Check sheet for the modelled part. Datum: model origin and axes. Units: mm. Face numbers are marked on the shaded views. A direction names the side the tool comes from. Coordinates: 2 decimals unless noted, no trailing zeros. Write each loop counter-clockwise with the first axis right and the second up, starting at its lowest first coordinate (ties: lowest second). Pieces come first, ordered by that corner, then holes. Notation, with made-up numbers: M -15,-4.5 L -10,-4.5 A17 cw -10,7.5 Z; hole C -32.5,9.5 d2. An arc over 180 degrees is marked long. Answer as CSV lines item,"result". Start each with the question number.
Q1. Sectioned sample at C-C, the plane x = -5. Record the cut outline in (y, z) (3 decimals), then the cut area to 3 significant figures.
Q2. Sectioned sample at A-A, the plane y = 10.75. Record the cut outline in (x, z) (1 decimal).
Q3. Depth check by flat-ended pin: pin 1 Ø2.5 at (x, y) = (33, 9.5) entering from -Z; pin 2 Ø3.5 at (x, z) = (-33.5, 1) entering from -Y; pin 3 Ø3 at (x, z) = (-20, 2) entering from +Y (3 decimals); pin 4 Ø2.5 at (y, z) = (10, 0) entering from -X. Enter the tip coordinate at first touch or a pass-through.
Q4. Mould release check, pull along X, two halves, no side actions. Record for the marked faces 1 and 2: pulls with the +X half, pulls with the -X half, needs draft (parallel to the pull), parting line crosses it, or undercut.
Q5. Thickness scan on line 1 along X through (y, z) = (7.5, 0); line 2 along Y through (x, z) = (20, -2.5) (3 decimals); line 3 along X through (y, z) = (4.25, -2.5). Record the ranges inside material, lowest first. Write a range as from..to.
Q6. Access from +Z, -Z, +X, -X, +Y, -Y to the whole of each face (thin tool, end or side, straight path). Record for the marked faces 3 and 4.
from build123d import *

# Parameters (mm, degrees)
SKETCH1_W            = 70.485
SKETCH1_H            = 6.35
BOSS_EXTRUDE1_DEPTH  = 3.175
SKETCH2_R            = 3.048
BOSS_EXTRUDE2_DEPTH  = 3.81
SKETCH3_W            = 6.096
SKETCH3_H            = 6.096
BOSS_EXTRUDE3_DEPTH  = 5.969
FILLET1_R            = 3.175
FILLET2_R            = 0.635
FILLET2_OF_MIRROR1_R = 0.635


with BuildPart() as part:
    # Sketch1 → Boss-Extrude1 (new body)
    with BuildSketch(Plane(origin=(0, 0, 0), x_dir=(1, 0, 0), z_dir=(0, 1, 0))):
        Rectangle(SKETCH1_W, SKETCH1_H)
    extrude(amount=BOSS_EXTRUDE1_DEPTH)

    # Sketch2 → Boss-Extrude2 (add)
    with BuildSketch(Plane(origin=(0, 3.175, 0), x_dir=(1, 0, 0), z_dir=(0, 1, 0))):
        with Locations(Location((32.0675, 0, 0), (0, 0, 90))):
            Circle(SKETCH2_R)
    boss_extrude2 = extrude(amount=BOSS_EXTRUDE2_DEPTH)

    # Sketch3 → Boss-Extrude3 (add)
    with BuildSketch(Plane(origin=(0, 6.985, 0), x_dir=(1, 0, 0), z_dir=(0, 1, 0))):
        with Locations((32.0675, 0)):
            Rectangle(SKETCH3_W, SKETCH3_H)
    boss_extrude3 = extrude(amount=BOSS_EXTRUDE3_DEPTH)

    # Fillet1
    fillet1_edges = [part.edges().sort_by_distance(p)[0] for p in [
        (-35.2425, 1.5875, 3.175),
        (-35.2425, 1.5875, -3.175),
        (35.2425, 1.5875, 3.175),
        (35.2425, 1.5875, -3.175),
    ]]
    fillet(fillet1_edges, radius=FILLET1_R - 0.0001)  # a hair under: the kernel refuses the full size

    # Fillet2
    fillet2_edges = [part.edges().sort_by_distance(p)[0] for p in [
        (35.1155, 9.9695, 3.048),
        (35.1155, 9.9695, -3.048),
        (29.0195, 9.9695, -3.048),
        (29.0195, 9.9695, 3.048),
    ]]
    fillet(fillet2_edges, radius=FILLET2_R)

    # Mirror1: Boss-Extrude2, Boss-Extrude3 across plane
    add(boss_extrude2.mirror(Plane(origin=(0, 0, 0), x_dir=(0, 0, 1), z_dir=(1, 0, 0))))
    add(boss_extrude3.mirror(Plane(origin=(0, 0, 0), x_dir=(0, 0, 1), z_dir=(1, 0, 0))))

    # Fillet2 of Mirror1
    fillet2_of_mirror1_edges = [part.edges().sort_by_distance(p)[0] for p in [
        (-35.1155, 9.9695, 3.048),
        (-35.1155, 9.9695, -3.048),
        (-29.0195, 9.9695, -3.048),
        (-29.0195, 9.9695, 3.048),
    ]]
    fillet(fillet2_of_mirror1_edges, radius=FILLET2_OF_MIRROR1_R)


solid = part.part
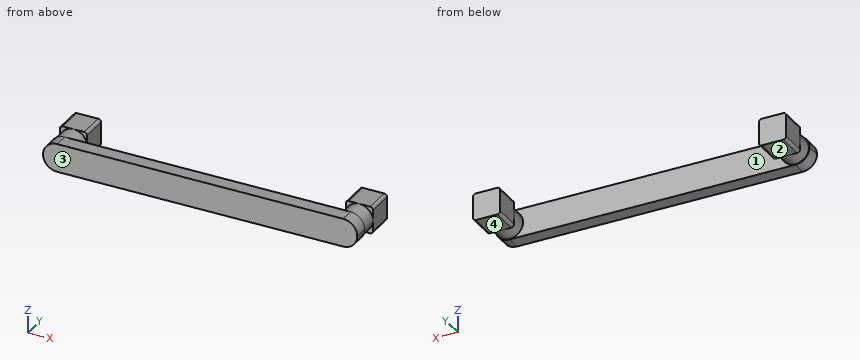
Output:
1,outline,"M 0,-3.175 L 3.175,-3.175 L 3.175,3.175 L 0,3.175 Z"
1,area,"20.2 mm^2"
2,outline,"M -35.1,-2.4 A0.6 ccw -34.5,-3 L -29.7,-3 A0.6 ccw -29,-2.4 L -29,2.4 A0.6 ccw -29.7,3 L -34.5,3 A0.6 ccw -35.1,2.4 Z; M 29,-2.4 A0.6 ccw 29.7,-3 L 34.5,-3 A0.6 ccw 35.1,-2.4 L 35.1,2.4 A0.6 ccw 34.5,3 L 29.7,3 A0.6 ccw 29,2.4 Z"
3,pin 1,"stops at z = -3.05"
3,pin 2,"stops at y = 0"
3,pin 3,"stops at y = 3.175"
3,pin 4,"stops at x = -35.12"
4,face 1,"undercut"
4,face 2,"needs draft"
5,line 1,"x = -35.12..-29.02, 29.02..35.12"
5,line 2,"y = 0..3.175"
5,line 3,"x = -33.81..-30.32, 30.32..33.81"
6,face 3,"+Z, -Z, +X, -X, -Y"
6,face 4,"-Z, +X, -X, +Y"
